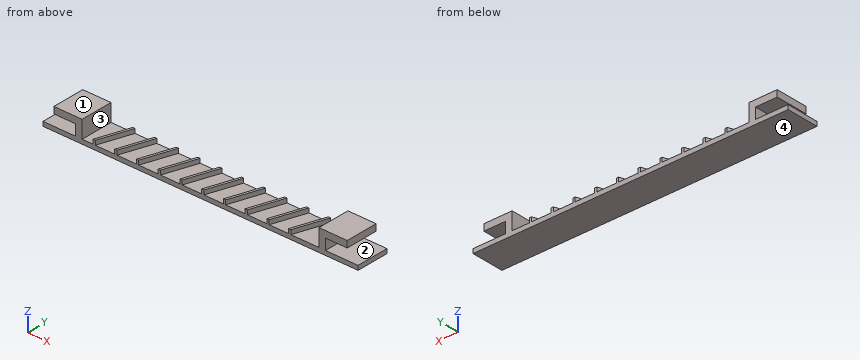
from build123d import *

# Parameters (mm, degrees)
F0_W     = 145
F0_H     = 15
F1_DEPTH = 2
F3_DEPTH = 15
F5_DEPTH = 2


with BuildPart() as f1:
    # F0 (on Top) → F1 (new body)
    with BuildSketch(Plane.XY):
        Rectangle(F0_W, F0_H)
    extrude(amount=F1_DEPTH)

    # F2 (on face) → F3 (join, through all)
    with BuildSketch(Plane.XZ.offset(7.5)):
        Polygon((-57.5, 7), (-57.5, 2), (-54.5, 2), (-54.5, 10), (-67.5, 10), (-67.5, 7), align=None)
        Polygon((57.5, 7), (67.5, 7), (67.5, 10), (54.5, 10), (54.5, 2), (57.5, 2), align=None)
    extrude(amount=-F3_DEPTH)

    # F4 (on face) → F5 (join)
    with BuildSketch(Plane.XY.offset(2)):
        Polygon((-44.5, 7.5), (-49.5, -7.5), (-48.445907, -7.5), (-43.445907, 7.5), align=None)
        Polygon((-34.5, 7.5), (-39.5, -7.5), (-38.445907, -7.5), (-33.445907, 7.5), align=None)
        Polygon((-24.5, 7.5), (-29.5, -7.5), (-28.445907, -7.5), (-23.445907, 7.5), align=None)
        Polygon((-14.5, 7.5), (-19.5, -7.5), (-18.445907, -7.5), (-13.445907, 7.5), align=None)
        Polygon((-4.5, 7.5), (-9.5, -7.5), (-8.445907, -7.5), (-3.445907, 7.5), align=None)
        Polygon((5.5, 7.5), (0.5, -7.5), (1.554093, -7.5), (6.554093, 7.5), align=None)
        Polygon((15.5, 7.5), (10.5, -7.5), (11.554093, -7.5), (16.554093, 7.5), align=None)
        Polygon((25.5, 7.5), (20.5, -7.5), (21.554093, -7.5), (26.554093, 7.5), align=None)
        Polygon((35.5, 7.5), (30.5, -7.5), (31.554093, -7.5), (36.554093, 7.5), align=None)
        Polygon((45.5, 7.5), (40.5, -7.5), (41.554093, -7.5), (46.554093, 7.5), align=None)
    extrude(amount=F5_DEPTH)


solid = f1.part
The listing builds one solid part. Answer for the finished solid, in the listing's coordinates (mm). Face numbers are marked on the shaded views. A direction names the side the tool comes from. Round coordinates to 2 decimals unless told otherwise and drop trailing zeros. Order: outer loops, then holes, each group sorted by start corner. A loop starts at its lowest first (then second) coordinate and runs counter-clockwise, first axis right, second up. Notation, with made-up numbers: (38.5, 79) -> (94.5, 79) arc R18 ccw to (94.5, 87) -> close; hole circle Ø2 at (52, -10.75). An arc over 180 degrees is marked (long way). Put each result on its own line as item: value.
Q1. Determine the mould class of the marked faces 3 and 4 for opening direction X: pulls with the +X half, pulls with the -X half, needs draft (parallel to the pull), parting line crosses it, or undercut.
Results list:
face 3: undercut
face 4: needs draft
Q2. Section B-B, the plane x = -51.5 is taken. Write down the section's boundary in (y, z).
Results list:
outline: (-7.5, 0) -> (7.5, 0) -> (7.5, 2) -> (-7.5, 2) -> close
Q3. Section A-A, the plane z = 8.25 is taken. Write down the section's boundary in (x, y), and give its area (3 significant figures).
Results list:
outline: (-67.5, -7.5) -> (-54.5, -7.5) -> (-54.5, 7.5) -> (-67.5, 7.5) -> close; (54.5, -7.5) -> (67.5, -7.5) -> (67.5, 7.5) -> (54.5, 7.5) -> close
area: 390 mm^2
Q4. Which of the six approach directions +Z, -Z, +X, -X, +Y, -Y give full straight-line access (tool end or side, diameter ignored) to the marked faces 1 and 2?
Results list:
face 1: +Z, +X, -X, +Y, -Y
face 2: +X, +Y, -Y
Q5. Each of these flat-tipped pins is pushed along its axis until it touches: P1, Ø1.5, axis at y = 0, z = 4, coming from the -X side; P2, Ø5, axis at x = -15, y = 2.5, coming from the +Z side; P3, Ø4, axis at x = -39.5, y = 2, coming from the +Z side. Where does it stop, or does it pass through?
Results list:
P1: x = -57.5
P2: z = 4
P3: z = 2
Q6. Consider line 1 along Z through (x, y) = (-60, -6.25); line 2 along X through (y, z) = (-4.5, 8.25); line 3 along X through (y, z) = (0.75, 5.25). Determine where each line is inside the solid, lowest interval first.
Results list:
line 1: 0 to 2, 7 to 10
line 2: -67.5 to -54.5, 54.5 to 67.5
line 3: -57.5 to -54.5, 54.5 to 57.5
